Geometry check sheet. Reference: the model listing, model coordinates, mm. A direction names the side the tool comes from. Coordinates: 2 decimals unless noted, no trailing zeros. Order: outer loops, then holes, each group sorted by start corner. A loop starts at its lowest first (then second) coordinate and runs counter-clockwise, first axis right, second up. Notation, with made-up numbers: (85.5, 36) - (103.5, 36) arc R14 ccw to (103.5, 53) - close; hole circle Ø6 at (52, 37). An arc over 180 degrees is marked (long way). Use CSV: the item, a comma, the result in double quotes. Start each with the question number.
1) Draft check along Y on faces 6 (the flat face through (0, 19, 5)), 7 (the flat face through (0, 66.373, 0)), 8 (the flat face through (-3.5, -6, 0)), 9 (the flat face through (3.7, 6.1, 0)). Enter one of: released by +Y, released by -Y, zero draft, split by the parting line, or undercut.
2) Depth check by flat-ended pin: P1, Ø6, axis at x = 4, y = 33.5, coming from the -Z side; P2, Ø6, axis at x = -4, y = 32.5, coming from the +Z side. Enter the tip coordinate at first touch or a pass-through.
3) Sectioned sample at A-A, the plane z = -2.5. Record the cut outline in (x, y).
4) Sectioned sample at B-B, the plane y = 41. Record the cut outline in (x, z), and give its area (3 significant figures).
5) Tool access check on faces 1 (the flat face through (4, 46, 0)), 2 (the flat face through (-7.5, 59, 0)), 3 (the flat face through (7.5, -20, 0)), 4 (the flat face through (-4, 7, 0)), 5 (the flat face through (-3, 45, 0)). Record the directions out of +Z, -Z, +X, -X, +Y, -Y that give a thin tool (end or side, any length) a straight path to the whole face; none if there is none.
6) Thickness scan on probe 1 along Y at (x, z) = (1.5, 2.75); probe 2 along Y at (x, z) = (-3.75, 3.75); probe 3 along Y at (x, z) = (6.75, 0.5). Record the ranges inside material, lowest first. Write a range as [from, to].
7) Sectioned sample at C-C, the plane x = -5.25. Record the cut outline in (y, z), and give its area (3 significant figures).
from build123d import *

# Parameters (mm, degrees)
SKETCH1_W           = 15
SKETCH1_H           = 15
BOSS_EXTRUDE1_DEPTH = 5
BOSS_EXTRUDE2_START = 5
BOSS_EXTRUDE2_DEPTH = 5
BOSS_EXTRUDE3_START = -5
BOSS_EXTRUDE3_DEPTH = 5
SKETCH1_5_W         = 15
SKETCH1_5_H         = 15
BOSS_EXTRUDE4_DEPTH = 5


with BuildPart() as part:
    # Sketch1 → Boss-Extrude1 (new, symmetric)
    with BuildSketch(Plane.XY):
        with Locations((0, -19.624355653)):
            Rectangle(SKETCH1_W, SKETCH1_H)
    boss_extrude1 = extrude(amount=BOSS_EXTRUDE1_DEPTH, both=True)

    # Sketch1<3> → Boss-Extrude2 (add)
    with BuildSketch(Plane.XY.offset(BOSS_EXTRUDE2_START)):
        Polygon((-6.5, -12.124355653), (0, -0.866025404), (-0.5, 0), (-7.5, -12.124355653), align=None)
        Polygon((0.5, 0), (7.5, 12.124355653), (6.5, 12.124355653), (0, 0.866025404), align=None)
        Polygon((0, -0.866025404), (0.5, 0), (0, 0.866025404), (-0.5, 0), align=None)
    boss_extrude2 = extrude(amount=-BOSS_EXTRUDE2_DEPTH)

    # Sketch1<4> → Boss-Extrude3 (add)
    with BuildSketch(Plane.XY.offset(BOSS_EXTRUDE3_START)):
        Polygon((0, 0.866025404), (-6.5, 12.124355653), (-7.5, 12.124355653), (-0.5, 0), align=None)
        Polygon((7.5, -12.124355653), (0.5, 0), (0, -0.866025404), (6.5, -12.124355653), align=None)
        Polygon((0, -0.866025404), (0.5, 0), (0, 0.866025404), (-0.5, 0), align=None)
    boss_extrude3 = extrude(amount=BOSS_EXTRUDE3_DEPTH)

    # Sketch1<5> → Boss-Extrude4 (add, symmetric)
    with BuildSketch(Plane.XY):
        with Locations((0, 19.624355653)):
            Rectangle(SKETCH1_5_W, SKETCH1_5_H)
    extrude(amount=BOSS_EXTRUDE4_DEPTH, both=True)

    # Mirror2: Boss-Extrude2, Boss-Extrude3 across plane
    add(boss_extrude2.mirror(Plane(origin=(0, 19.624355653, 0), x_dir=(0, 0, 1), z_dir=(0, -1, 0))))
    add(boss_extrude3.mirror(Plane(origin=(0, 19.624355653, 0), x_dir=(0, 0, 1), z_dir=(0, -1, 0))))

    # Mirror3: Boss-Extrude1 across plane
    add(boss_extrude1.mirror(Plane(origin=(0, 19.624355653, 0), x_dir=(0, 0, 1), z_dir=(0, -1, 0))))


solid = part.part
Evaluation:
1,face 6,"zero draft"
1,face 7,"released by +Y"
1,face 8,"undercut"
1,face 9,"undercut"
2,P1,"z = 0"
2,P2,"z = 0"
3,outline,"(-7.5, -27.12) - (7.5, -27.12) - (7.5, -12.12) - (-6.5, 12.12) - (7.5, 12.12) - (7.5, 27.12) - (-6.5, 27.12) - (7.5, 51.37) - (7.5, 66.37) - (-7.5, 66.37) - (-7.5, 51.37) - (6.5, 51.37) - (-7.5, 27.12) - (-7.5, 12.12) - (6.5, -12.12) - (-7.5, -12.12) - close"
4,outline,"(-1.51, 0) - (-0.51, 0) - (-0.51, 5) - (-1.51, 5) - close; (0.51, -5) - (1.51, -5) - (1.51, 0) - (0.51, 0) - close"
4,area,"10.0 mm²"
5,face 1,"+Z, +X"
5,face 2,"+Z, -Z, -X, +Y, -Y"
5,face 3,"+Z, -Z, +X, +Y, -Y"
5,face 4,"+Z, -X"
5,face 5,"-Z, -X"
6,probe 1,"[-27.12, -12.12], [1.73, 3.46], [12.12, 27.12], [35.78, 37.52], [51.37, 66.37]"
6,probe 2,"[-27.12, -12.12], [-7.36, -5.63], [12.12, 27.12], [44.88, 46.61], [51.37, 66.37]"
6,probe 3,"[-27.12, -12.12], [10.83, 28.42], [51.37, 66.37]"
7,outline,"(-27.12, -5) - (-12.12, -5) - (-12.12, 5) - (-27.12, 5) - close; (-9.96, 0) - (-8.23, 0) - (-8.23, 5) - (-9.96, 5) - close; (8.23, -5) - (9.96, -5) - (9.96, 0) - (8.23, 0) - close; (12.12, -5) - (27.12, -5) - (27.12, 5) - (12.12, 5) - close; (29.29, -5) - (31.02, -5) - (31.02, 0) - (29.29, 0) - close; (47.48, 0) - (49.21, 0) - (49.21, 5) - (47.48, 5) - close; (51.37, -5) - (66.37, -5) - (66.37, 5) - (51.37, 5) - close"
7,area,"485 mm²"
